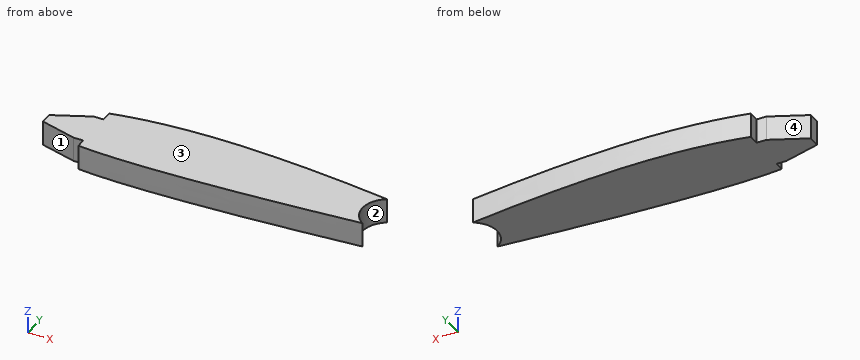
Autodesk Inventor part; units mm, degrees
ref_plane "YZ Plane" through (0, 0, 0) normal (1, 0, 0) x (0, 1, 0)
ref_plane "XZ Plane" through (0, 0, 0) normal (0, 1, 0) x (-1, 0, 0)
ref_plane "XY Plane" through (0, 0, 0) normal (0, 0, 1) x (1, 0, 0)
sketch "Sketch2" plane through (0, 0, 0) normal (0, 0, 1) x (1, 0, 0)
  spline S0 degree 5 poles (319.6498, 0.0573) (319.6501, 0.0612) (319.6024, 0.0717) (319.3745, 0.1032) (319.3587, 0.1577) (318.7204, 0.2502) (318.4411, 0.3675) (317.6227, 0.5236) (316.9347, 0.7102) (315.9239, 0.9334) (314.8763, 1.1861) (313.6258, 1.4728) (312.2675, 1.7887) (310.7514, 2.1347) (309.1071, 2.5099) (307.3204, 2.9131) (305.4017, 3.3421) (303.3481, 3.7974) (301.1639, 4.2757) (298.8502, 4.7782) (296.4092, 5.301) (293.8432, 5.8446) (291.1548, 6.4061) (288.3466, 6.9857) (285.4207, 7.5803) (282.3807, 8.1894) (279.2284, 8.8107) (275.968, 9.4437) (272.6016, 10.0865) (269.1329, 10.7361) (265.5656, 11.3942) (261.9019, 12.0551) (258.1469, 12.7207) (254.3029, 13.3883) (250.3742, 14.0555) (246.3647, 14.7217) (242.2776, 15.3854) (238.118, 16.0441) (233.8887, 16.6979) (229.5952, 17.3434) (225.2402, 17.981) (220.8297, 18.6074) (216.3658, 19.2226) (211.8552, 19.8242) (207.3009, 20.4107) (202.7077, 20.9813) (198.0804, 21.5339) (193.4232, 22.0679) (188.7413, 22.58) (184.0389, 23.0713) (179.321, 23.5382) (174.592, 23.982) (169.8567, 24.3971) (165.1201, 24.7874) (160.3872, 25.1472) (155.6604, 25.4776) (150.948, 25.7772) (146.2454, 26.0449) (141.5744, 26.278) (136.9015, 26.4795) (132.2479, 26.6311) (127.6319, 26.7393) (123.054, 26.7999) (118.5202, 26.8147) (114.0397, 26.7815) (109.6094, 26.7031) (105.2517, 26.5723) (100.9331, 26.4088) (96.7495, 26.1663) (92.5147, 25.9483) (88.6376, 25.5343) (84.2302, 25.3974) (81.2071, 24.5612) (76.5297, 24.5259) (73.18, 23.8676) (69.3619, 23.413) (65.9721, 22.8018) (62.3454, 22.244) (59.4319, 21.514) (55.4307, 21.0148) (53.2464, 20.1084) (49.5889, 19.537) (47.2944, 18.6473) (44.3884, 17.909) (41.914, 17.071) (39.4431, 16.2394) (37.1538, 15.3738) (34.9769, 14.4941) (32.9455, 13.5944) (31.0501, 12.6807) (29.2961, 11.7542) (27.6837, 10.8151) (26.2149, 9.8673) (24.8895, 8.9103) (23.7099, 7.9467) (22.6751, 6.976) (21.7868, 6.0004) (21.0458, 5.0186) (20.4526, 4.032) (20.0117, 3.0392) (19.7221, 2.0438) (19.5893, 1.0479) (19.6118, 0.0538) (19.7865, -0.9258) (20.1138, -1.8742) (20.591, -2.7944) (21.2165, -3.6796) (21.9855, -4.5321) (22.8956, -5.3514) (23.9453, -6.1385) (25.1332, -6.8944) (26.4582, -7.6188) (27.9184, -8.3123) (29.5136, -8.9751) (31.2409, -9.6071) (33.0997, -10.2067) (35.0892, -10.7758) (37.2002, -11.3131) (39.4562, -11.8174) (41.7927, -12.2939) (44.3651, -12.7275) (46.7744, -13.1584) (50.0005, -13.481) (52.1533, -13.8927) (55.9371, -14.1294) (58.2153, -14.4717) (61.732, -14.6854) (64.8012, -14.9153) (68.2287, -15.092) (71.6338, -15.2498) (75.1915, -15.3722) (78.8138, -15.4692) (82.5326, -15.5359) (86.3291, -15.5764) (90.2061, -15.5901) (94.1575, -15.5787) (98.1812, -15.5438) (102.2727, -15.4851) (106.4286, -15.4059) (110.6456, -15.3062) (114.9188, -15.1867) (119.2459, -15.0512) (123.6218, -14.8988) (128.0442, -14.7319) (132.5111, -14.552) (137.0141, -14.3592) (141.5621, -14.1606) (146.1675, -13.9403) (150.787, -13.7052) (155.434, -13.4523) (160.0951, -13.1857) (164.7676, -12.9046) (169.4465, -12.6129) (174.1261, -12.3082) (178.8033, -11.9955) (183.4722, -11.6727) (188.1294, -11.3426) (192.7696, -11.0072) (197.3886, -10.6641) (201.9818, -10.3188) (206.5448, -9.9678) (211.0728, -9.6157) (215.5623, -9.2611) (220.0069, -8.9047) (224.4048, -8.5497) (228.7492, -8.193) (233.0373, -7.8393) (237.2647, -7.4865) (241.4259, -7.1353) (245.5189, -6.7884) (249.5374, -6.4441) (253.4791, -6.104) (257.3389, -5.7683) (261.1136, -5.4376) (264.7987, -5.113) (268.3914, -4.7937) (271.8871, -4.4807) (275.2826, -4.1749) (278.5752, -3.8759) (281.7596, -3.585) (284.8354, -3.3021) (287.7962, -3.0278) (290.6419, -2.763) (293.3672, -2.5063) (295.9712, -2.2616) (298.4496, -2.0246) (300.8012, -1.801) (303.0222, -1.5859) (305.1122, -1.3849) (307.0656, -1.194) (308.8864, -1.0166) (310.5623, -0.8504) (312.1091, -0.6993) (313.4945, -0.5587) (314.7717, -0.4371) (315.8415, -0.3205) (316.8737, -0.2329) (317.5782, -0.1363) (318.4119, -0.0906) (318.7016, -0.0103) (319.3493, -0.0034) (319.3699, 0.0485) (319.6005, 0.0494) (319.6495, 0.0534) (319.6498, 0.0573) knots 0 0 0 0 0 0 0.001406 0.002637 0.004353 0.006443 0.008834 0.011487 0.014375 0.017478 0.020781 0.02427 0.027934 0.031762 0.035746 0.039878 0.044151 0.048559 0.053094 0.057751 0.062526 0.067412 0.072404 0.077499 0.082692 0.087977 0.093351 0.098811 0.104351 0.109968 0.115658 0.121418 0.127243 0.133131 0.139077 0.145079 0.151132 0.157233 0.163379 0.169567 0.175793 0.182054 0.188346 0.194667 0.201013 0.20738 0.213767 0.220168 0.226582 0.233004 0.239433 0.245864 0.252294 0.258721 0.265141 0.27155 0.27795 0.284339 0.290715 0.297074 0.303413 0.309725 0.316005 0.32225 0.328456 0.33462 0.340739 0.34681 0.352829 0.358735 0.364639 0.370482 0.376261 0.381971 0.38767 0.393236 0.398773 0.404177 0.409526 0.414755 0.419891 0.424884 0.429828 0.434638 0.439375 0.444 0.448512 0.452907 0.457182 0.461332 0.465356 0.469251 0.473017 0.476652 0.480158 0.48354 0.486805 0.489964 0.493033 0.496034 0.498989 0.501921 0.504852 0.507807 0.510807 0.513873 0.517028 0.520286 0.523658 0.527152 0.530771 0.534516 0.538388 0.542384 0.546503 0.550741 0.555095 0.559563 0.56414 0.568856 0.57364 0.578576 0.583553 0.588622 0.593747 0.598989 0.604262 0.609667 0.615146 0.620698 0.626318 0.632003 0.637751 0.643558 0.649421 0.655338 0.661304 0.667318 0.673375 0.679474 0.685611 0.691783 0.697987 0.704223 0.710491 0.716788 0.723111 0.729457 0.73582 0.742195 0.748576 0.754963 0.761351 0.767737 0.774118 0.780492 0.786854 0.793202 0.799533 0.805843 0.812129 0.818388 0.824617 0.830812 0.836971 0.843089 0.849164 0.855191 0.861169 0.867092 0.872959 0.878764 0.884505 0.890178 0.895778 0.901303 0.906749 0.91211 0.917384 0.922566 0.927651 0.932635 0.937513 0.942281 0.946932 0.951462 0.955865 0.960134 0.964263 0.968244 0.97207 0.975732 0.979219 0.982521 0.985624 0.988511 0.991164 0.993554 0.995643 0.997359 0.998591 1 1 1 1 1 1
  line L0 (79.5135, 4.6359) -> (79.5135, 24.6083) construction
  line L1 (79.5135, 4.6359) -> (209.6498, 4.6359) construction
  line L2 (319.6498, 0.0573) -> (219.6498, 0.0573) construction
  line L3 (219.6499, 18.7671) -> (219.6499, -8.9327) construction
  line L4 (28.0055, 4.5054) -> (28.0055, -2.4946)
  line L5 (19.627, 1.0326) -> (319.6498, 0.0573) construction
  line L6 (49.7105, 14.4213) -> (55.6079, 14.4213)
  line L7 (49.7104, -8.4915) -> (55.6078, -8.4915)
  line L8 (28.0055, 4.5054) -> (49.7105, 14.4213)
  line L9 (28.0055, -2.4946) -> (49.7104, -8.4915)
  line L10 (55.6079, 14.4213) -> (55.6079, 20.8726)
  line L11 (55.6078, -8.4915) -> (55.6078, -14.1513)
  arc A0 (225.2869, 17.9694) -> (224.4503, -8.5446) centre (233.3969, 4.4433) ccw
  point P0 (0, 0)
  point P1 (319.3573, 0.1272)
  point P2 (318.9918, 0.2142)
  point P3 (318.4802, 0.3354)
  point P4 (317.8238, 0.4911)
  point P5 (317.0222, 0.6801)
  point P6 (316.0769, 0.9024)
  point P7 (314.9885, 1.1568)
  point P8 (313.7582, 1.443)
  point P9 (312.3866, 1.7598)
  point P10 (310.8752, 2.1063)
  point P11 (309.2258, 2.4819)
  point P12 (307.4393, 2.8854)
  point P13 (305.5178, 3.3153)
  point P14 (303.4628, 3.7707)
  point P15 (301.2764, 4.2501)
  point P16 (298.9607, 4.7526)
  point P17 (296.5175, 5.2764)
  point P18 (293.9492, 5.8203)
  point P19 (291.2585, 6.3828)
  point P20 (288.4478, 6.9627)
  point P21 (285.5195, 7.5582)
  point P22 (282.4766, 8.1678)
  point P23 (279.3218, 8.79)
  point P24 (276.0584, 9.4236)
  point P25 (272.6891, 10.0668)
  point P26 (269.2175, 10.7178)
  point P27 (265.6469, 11.3757)
  point P28 (261.9803, 12.0381)
  point P29 (258.2219, 12.7041)
  point P30 (254.3747, 13.3722)
  point P31 (250.4426, 14.0403)
  point P32 (246.4295, 14.7072)
  point P33 (242.339, 15.3714)
  point P34 (238.1756, 16.0311)
  point P35 (233.9428, 16.6851)
  point P36 (229.6454, 17.3316)
  point P37 (220.8723, 18.5967)
  point P38 (216.4049, 19.2123)
  point P39 (211.8901, 19.8144)
  point P40 (207.332, 20.4015)
  point P41 (202.7347, 20.9724)
  point P42 (198.1034, 21.5256)
  point P43 (193.4423, 22.0596)
  point P44 (188.7563, 22.5726)
  point P45 (184.0499, 23.0637)
  point P46 (179.3279, 23.5314)
  point P47 (174.5948, 23.9745)
  point P48 (169.8554, 24.3909)
  point P49 (165.1148, 24.7803)
  point P50 (160.3775, 25.1406)
  point P51 (155.6479, 25.4709)
  point P52 (150.9316, 25.7703)
  point P53 (146.233, 26.0373)
  point P54 (141.557, 26.2707)
  point P55 (136.882, 26.4681)
  point P56 (132.2209, 26.6211)
  point P57 (127.5964, 26.7282)
  point P58 (123.0133, 26.7888)
  point P59 (118.4761, 26.8026)
  point P60 (113.9902, 26.7693)
  point P61 (109.5601, 26.6886)
  point P62 (105.191, 26.5611)
  point P63 (100.8866, 26.3866)
  point P64 (96.6524, 26.1647)
  point P65 (92.4927, 25.8975)
  point P66 (88.4121, 25.5832)
  point P67 (84.4152, 25.2282)
  point P68 (80.9052, 24.7441)
  point P69 (76.6873, 24.3761)
  point P70 (72.9635, 23.8905)
  point P71 (69.3402, 23.3611)
  point P72 (65.8208, 22.7938)
  point P73 (62.4086, 22.1883)
  point P74 (59.107, 21.5464)
  point P75 (52.8493, 20.1606)
  point P76 (49.7105, 19.4213)
  point P77 (47.0737, 18.6507)
  point P78 (44.3741, 17.8542)
  point P79 (41.8034, 17.0322)
  point P80 (39.3638, 16.1874)
  point P81 (37.0583, 15.3213)
  point P82 (34.8884, 14.4363)
  point P83 (32.8568, 13.534)
  point P84 (30.965, 12.6166)
  point P85 (29.2145, 11.686)
  point P86 (27.6071, 10.7437)
  point P87 (26.1443, 9.7921)
  point P88 (24.8269, 8.8324)
  point P89 (23.6566, 7.8664)
  point P90 (22.6336, 6.8953)
  point P91 (21.7591, 5.9209)
  point P92 (21.0334, 4.9441)
  point P93 (20.4571, 3.9661)
  point P94 (20.0308, 2.9875)
  point P95 (19.7539, 2.0098)
  point P96 (19.6496, 0.0573)
  point P97 (19.8205, -0.9033)
  point P98 (20.1376, -1.8357)
  point P99 (20.6002, -2.7402)
  point P100 (21.208, -3.6159)
  point P101 (21.9598, -4.4628)
  point P102 (22.8544, -5.2806)
  point P103 (23.8909, -6.069)
  point P104 (25.0681, -6.8277)
  point P105 (26.3846, -7.5561)
  point P106 (27.8384, -8.2539)
  point P107 (29.4284, -8.9211)
  point P108 (31.1522, -9.5571)
  point P109 (33.0086, -10.1613)
  point P110 (34.9949, -10.734)
  point P111 (37.1093, -11.2746)
  point P112 (39.3497, -11.7828)
  point P113 (41.7134, -12.2586)
  point P114 (44.198, -12.702)
  point P115 (46.8014, -13.1127)
  point P116 (49.7104, -13.4915)
  point P117 (52.3532, -13.8357)
  point P118 (58.3469, -14.4294)
  point P119 (61.5023, -14.6781)
  point P120 (64.7591, -14.8953)
  point P121 (68.1149, -15.0813)
  point P122 (71.5661, -15.237)
  point P123 (75.1094, -15.3627)
  point P124 (78.7418, -15.4596)
  point P125 (82.46, -15.528)
  point P126 (86.2607, -15.5691)
  point P127 (90.14, -15.5838)
  point P128 (94.0946, -15.5733)
  point P129 (98.1212, -15.5388)
  point P130 (102.2159, -15.4812)
  point P131 (106.3751, -15.4023)
  point P132 (110.5952, -15.303)
  point P133 (114.872, -15.1845)
  point P134 (119.2022, -15.0489)
  point P135 (123.5813, -14.8971)
  point P136 (128.006, -14.7306)
  point P137 (132.4718, -14.5509)
  point P138 (136.9748, -14.3598)
  point P139 (141.5285, -14.1576)
  point P140 (146.1365, -13.9383)
  point P141 (150.7679, -13.7022)
  point P142 (155.4191, -13.4499)
  point P143 (160.0853, -13.1829)
  point P144 (164.7617, -12.9024)
  point P145 (169.4444, -12.6099)
  point P146 (174.1283, -12.306)
  point P147 (178.8092, -11.9925)
  point P148 (183.4823, -11.67)
  point P149 (188.1434, -11.34)
  point P150 (192.7877, -11.0037)
  point P151 (197.4106, -10.6614)
  point P152 (202.0079, -10.3149)
  point P153 (206.5747, -9.9645)
  point P154 (211.1069, -9.6117)
  point P155 (215.5999, -9.2568)
  point P156 (220.0489, -8.9007)
  point P157 (228.7987, -8.1885)
  point P158 (233.0906, -7.8339)
  point P159 (237.3214, -7.4808)
  point P160 (241.4866, -7.1298)
  point P161 (245.5828, -6.7821)
  point P162 (249.6052, -6.4377)
  point P163 (253.5502, -6.0972)
  point P164 (257.4136, -5.7612)
  point P165 (261.1915, -5.4303)
  point P166 (264.88, -5.1051)
  point P167 (268.4758, -4.7856)
  point P168 (271.9747, -4.4724)
  point P169 (275.3734, -4.1661)
  point P170 (278.6686, -3.867)
  point P171 (281.8564, -3.5757)
  point P172 (284.9344, -3.2925)
  point P173 (287.8984, -3.018)
  point P174 (290.7463, -2.7525)
  point P175 (293.4745, -2.4963)
  point P176 (296.0806, -2.2503)
  point P177 (298.5616, -2.0142)
  point P178 (300.9151, -1.7892)
  point P179 (303.1387, -1.575)
  point P180 (305.23, -1.3728)
  point P181 (307.1866, -1.1823)
  point P182 (309.007, -1.0041)
  point P183 (310.6885, -0.8385)
  point P184 (312.2302, -0.6861)
  point P185 (313.6297, -0.5472)
  point P186 (314.8861, -0.4221)
  point P187 (315.9976, -0.3108)
  point P188 (316.9636, -0.2139)
  point P189 (317.7826, -0.1314)
  point P190 (318.4537, -0.0636)
  point P191 (318.9766, -0.0108)
  point P192 (319.3503, 0.027)
  point P193 (319.5743, 0.0498)
  point P194 (209.6498, 0.0573)
  point P195 (28.0055, 1.0054)
  point P196 (217.627, 4.6359)
  dimension "d2" = 300.0001
  dimension "d19" = 110
  dimension "d22" = 100
  dimension "d23" = 7
  dimension "d24" = 5
  dimension "d25" = 5
  dimension "d44" = 198
  dimension "d46" = 59.8865
extrude "Extrusion6" add sketch "Sketch2" along normal blind 15 contours A0 S0 L11 L7 L9 L4 L8 L6 L10
properties part number "2414 basic aerofoil" material "Polyurethane Foam"
Work out the finished part from the listing and answer in its coordinate system (mm). Face numbers are marked on the shaded views. Give positions to 0.01 mm unless a question says otherwise; leave off trailing zeros. Loops run counter-clockwise (first coordinate to the right, second up) from the corner with the lowest first, then second, coordinate; pieces in that order, holes last. Notation, with made-up numbers: M -11.5,19 L 22.5,19 A21 ccw 22.5,39 Z; hole C -16,-33 d3. An arc over 180 degrees is marked long. One line per item, written item: value. Start each with the question number.
1. Determine the mould class of the marked faces 1, 2, 3 and 4 for opening direction Y: released by +Y, released by -Y, zero draft, split by the parting line, or undercut.
2. Each of these flat-tipped pins is pushed along its axis until it touches: P1, Ø1.5, axis at x = 180.5, z = 7, coming from the -Y side; P2, Ø1, axis at y = 13.5, z = 3, coming from the -X side; P3, Ø4.5, axis at x = 53, z = 11, coming from the -Y side. Where does it stop, or does it pass through?
3. Find section A-A (y = -0.5). Give the vertices of the cut face in (x, z), and give its area (3 significant figures).
4. Find the intervals of material crossed by probe 1 along Y at (x, z) = (184.5, 4.75); probe 2 along X at (y, z) = (10, 6); probe 3 along Y at (x, z) = (122.5, 3), in increasing order.
Reported:
1. face 1: released by -Y
1. face 2: undercut
1. face 3: zero draft
1. face 4: released by +Y
2. P1: stops at y = -11.93
2. P2: stops at x = 46.6
2. P3: stops at y = -8.49
3. outline: M 28.01,0 L 218.42,0 L 218.42,15 L 28.01,15 Z
3. area: 2,860 mm²
4. probe 1: y = -11.6 to 23.02
4. probe 2: x = 40.03 to 218.64
4. probe 3: y = -14.94 to 26.79
